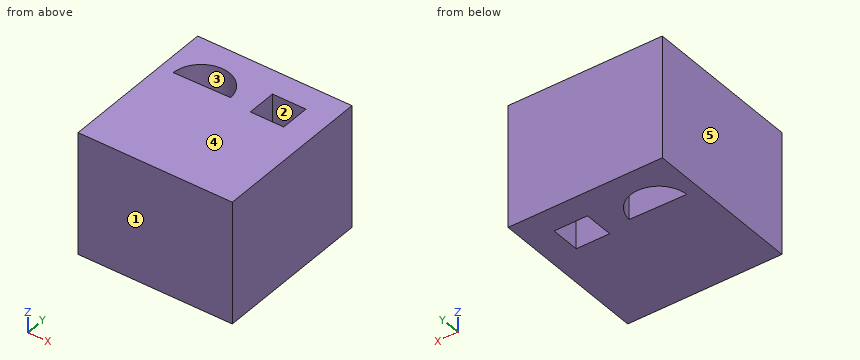
```python
from build123d import *

# Parameters (mm, degrees)
F0_W     = 64.047658
F0_H     = 66.427136
F1_DEPTH = 50.8
F2_W     = 13.880294
F2_H     = 12.293976
F3_DEPTH = 50.8
F5_DEPTH = 50.8


with BuildPart() as f1:
    # F0 (on Top) → F1 (new body)
    with BuildSketch(Plane.XY):
        with Locations((-1.487176, 3.172639)):
            Rectangle(F0_W, F0_H)
    extrude(amount=F1_DEPTH)

    # F2 (on face) → F3 (cut)
    with BuildSketch(Plane.XY.offset(50.8)):
        with Locations((12.492267, 19.531561)):
            Rectangle(F2_W, F2_H)
    extrude(amount=-F3_DEPTH, mode=Mode.SUBTRACT)

    # F4 (on face) → F5 (cut)
    with BuildSketch(Plane.XY.offset(50.8)):
        with BuildLine():
            Line((-27.958885, 15.367473), (-4.362379, 15.764052))
            ThreePointArc((-4.362379, 15.764052), (-16.350913, 26.887516), (-27.958885, 15.367473))
        make_face()
    extrude(amount=-F5_DEPTH, mode=Mode.SUBTRACT)


solid = f1.part
```
Model file for the job. Use its own axes, mm. Face numbers are marked on the shaded views. A direction names the side the tool comes from. Coordinates: 2 decimals unless noted, no trailing zeros. Order: outer loops, then holes, each group sorted by start corner. A loop starts at its lowest first (then second) coordinate and runs counter-clockwise, first axis right, second up. Notation, with made-up numbers: (-21, 64) - (32, 64) arc R21 cw to (32, 83) - close; hole circle Ø3 at (79, 60). An arc over 180 degrees is marked (long way). Return JSON: item names as keys, results as strings. Group by question number.
1) Saw through at A-A, the plane x = 18. Write the cut outline in (y, z), plus the area to 3 significant figures.
2) Saw through at B-B, the plane z = 20.5. Write the cut outline in (x, y), plus the area to 3 significant figures.
3) Saw through at C-C, the plane y = 18.5. Write the cut outline in (x, z).
4) Saw through at D-D, the plane x = -24.5. Write the cut outline in (y, z), plus the area to 3 significant figures.
5) Probe line 1 (Y direction, x = 16, z = 13); line 2 (X direction, y = 20, z = 8.5); line 3 (X direction, y = 24, z = 28). List the from-to ranges inside material, lowest first. Write a range as from..to.
6) Mould opens along X. For the marked faces 3, 4 and 5 say: released by +X, released by -X, zero draft, split by the parting line, or undercut.
7) Tool access for the marked faces 1 and 2: list every direction of +Z, -Z, +X, -X, +Y, -Y with a clear straight run to the whole face (end or side of a thin tool).
Values found:
{
 "1": {"outline": "(-30.04, 0) - (13.38, 0) - (13.38, 50.8) - (-30.04, 50.8) - close; (25.68, 0) - (36.39, 0) - (36.39, 50.8) - (25.68, 50.8) - close", "area": "2,750 mm²"},
 "2": {"outline": "(-33.51, -30.04) - (30.54, -30.04) - (30.54, 36.39) - (-33.51, 36.39) - close; hole (-27.96, 15.37) - (-4.36, 15.76) arc R11.81 ccw to start; hole (5.55, 13.38) - (19.43, 13.38) - (19.43, 25.68) - (5.55, 25.68) - close", "area": "3,880 mm²"},
 "3": {"outline": "(-33.51, 0) - (-27.46, 0) - (-27.46, 50.8) - (-33.51, 50.8) - close; (-4.85, 0) - (5.55, 0) - (5.55, 50.8) - (-4.85, 50.8) - close; (19.43, 0) - (30.54, 0) - (30.54, 50.8) - (19.43, 50.8) - close"},
 "4": {"outline": "(-30.04, 0) - (15.43, 0) - (15.43, 50.8) - (-30.04, 50.8) - close; (23.43, 0) - (36.39, 0) - (36.39, 50.8) - (23.43, 50.8) - close", "area": "2,970 mm²"},
 "5": {"line 1": "y = -30.04..13.38, 25.68..36.39", "line 2": "x = -33.51..-26.89, -5.42..5.55, 19.43..30.54", "line 3": "x = -33.51..-23.89, -8.41..5.55, 19.43..30.54"},
 "6": {"face 3": "undercut", "face 4": "zero draft", "face 5": "released by -X"},
 "7": {"face 1": "+Z, -Z, +X, -X, -Y", "face 2": "+Z, -Z"}
}
